Input: part model. Units: mm. Frame: model coordinates. A direction names the side the tool comes from. Round coordinates to 2 decimals unless told otherwise and drop trailing zeros. Write item = value, one per line.
```python
from build123d import *

# Parameters (mm, degrees)
F0_W           = 25.4
F0_H           = 19.05
F1_DEPTH       = 6.35
F3_DEPTH       = 6.351
F5_D           = 3.7973
F5_CSINK_D     = 7.7978
F5_CSINK_ANGLE = 82
F6_R           = 3.175


with BuildPart() as f1:
    # F0 (on Top) → F1 (new body)
    with BuildSketch(Plane.XY):
        Rectangle(F0_W, F0_H)
    extrude(amount=F1_DEPTH)

    # F2 (on face) → F3 (cut, through all)
    with BuildSketch(Plane.XY.offset(6.35)):
        with BuildLine():
            Line((4.1275, -9.525), (4.1275, 0))
            ThreePointArc((4.1275, 0), (0, 4.1275), (-4.1275, 0))
            Line((-4.1275, 0), (-4.1275, -9.525))
            Line((-4.1275, -9.525), (4.1275, -9.525))
        make_face()
    extrude(amount=-F3_DEPTH, mode=Mode.SUBTRACT)

    # F5 (through all)
    with Locations(Plane.XY.offset(6.35)):
        with Locations((-8.73125, 4.7625), (8.73125, 4.7625), (8.73125, -4.7625), (-8.73125, -4.7625)):
            CounterSinkHole(F5_D / 2, F5_CSINK_D / 2, counter_sink_angle=F5_CSINK_ANGLE)

    # F6
    f6_edges = [f1.edges().sort_by_distance(p)[0] for p in [
        (-12.7, 9.525, 3.175),
        (-12.7, -9.525, 3.175),
        (12.7, -9.525, 3.175),
        (12.7, 9.525, 3.175),
    ]]
    fillet(f6_edges, radius=F6_R)


solid = f1.part
```
1) Draft query along Y for faces 1 (the face through (9.1, 2.9, 2)), 2 (the face through (-12.7, 0, 3)), 3 (the face through (7, -9.525, 3)). Return one class per face: +Y half, -Y half, draft (parallel to the pull), parting line (faces both ways), or undercut.
Solutions:
face_1 = undercut
face_2 = draft
face_3 = -Y half
2) Cut plane A-A (z = 5.5). Count the separate pieces of the cut face and the enclosed holes in it, and give its area (3 significant figures).
Solutions:
separate_pieces = 1
enclosed_holes = 4
area = 244 mm^2
3) Line query: L1, parallel to X at y = -1, z = 5; L2, parallel to Y at x = -8.5, z = 2 (3 decimals); L3, parallel to X at y = 4.5, z = 2. Output: solid intervals per line, ascending. Write a range as from..to.
Solutions:
L1 = -12.7..-4.13, 4.13..12.7
L2 = -9.525..-6.647, -2.878..2.878, 6.647..9.525
L3 = -12.7..-10.61, -6.85..6.85, 10.61..12.7
4) First-contact query: P1, Ø8, axis at x = -6.5, y = -2, coming from the -Z side; P2, Ø4.5, axis at x = -8.73, y = -4.76, coming from the +Z side. Flat tips, straight axial feed; report the tip coordinate or a pass-through.
Solutions:
P1 = 0
P2 = 4.46
5) Access query for faces 4 (the face through (-1, 4.3, 6.35)), 5 (the face through (4.128, -5, 3)). Directions: +Z, -Z, +X, -X, +Y, -Y. A direction counts if a zero-diameter tool reaches every point of the face in a straight line with its end or side. Return the directions, or none.
Solutions:
face_4 = +Z, +X, -X, +Y, -Y
face_5 = +Z, -Z, -Y
